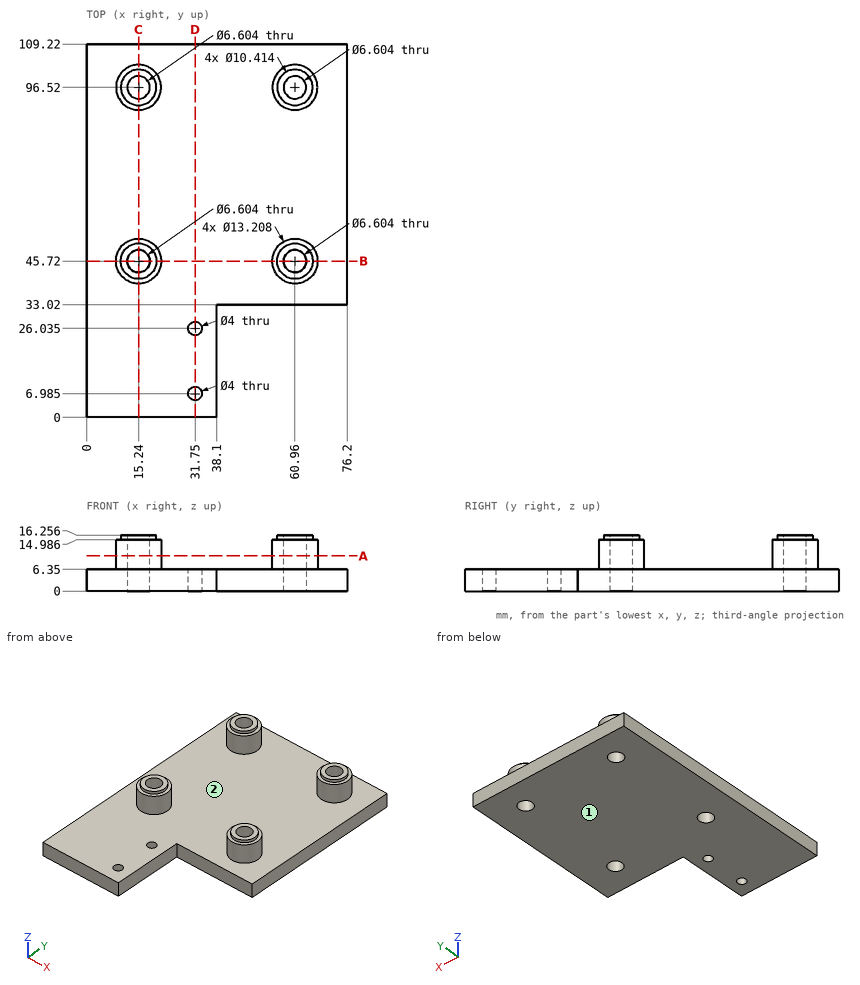
For this review, use the dimensioned drawing (mm, ordinates from the lowest corner) and the shaded views. Give positions to 0.01 mm unless a question says otherwise; leave off trailing zeros. Write each loop counter-clockwise with the first axis right and the second up, starting at its lowest first coordinate (ties: lowest second). Pieces come first, ordered by that corner, then holes. Notation, with made-up numbers: M 71,66 L 95,66 A27 ccw 95,88 Z; hole C -2.75,80 d11. An arc over 180 degrees is marked long. Answer as a JSON object with one key per item and string values. Group by question number.
1) For line 1 along Y through (x, z) = (60.96, 3.5); line 2 along Y through (x, z) = (60.96, 12.25); line 3 along X through (y, z) = (43.5, 4.25), list the stretches that pass through material, from the lowest coordinate up.
2) Mouldability with a two-part tool opening along Y and no side actions: class the marked faces 1 and 2 as released by +Y, released by -Y, zero draft, split by the parting line, or undercut.
3) Clearance check with flat-ended pins moving along their axes: pin 1 Ø6.5 at (x, y) = (31.75, 26.035) entering from +Z; pin 2 Ø8.5 at (x, y) = (60.96, 96.52) entering from -Z; pin 3 Ø8 at (x, z) = (60, 6.5) entering from -Y; pin 4 Ø7 at (y, z) = (17, 4) entering from +X. State where each tip first meets the part, or that it passes through.
4) We need section C-C (x = 15.24). Give the boundary of the cut face in (y, z).
5) We need section D-D (x = 31.75). Give the boundary of the cut face in (y, z) (3 decimals).
6) We need section B-B (y = 45.72). Give the boundary of the cut face in (x, z), and give its area (3 significant figures).
7) We need section A-A (z = 10.25). Give the boundary of the cut face in (x, y).
Answer key:
{
 "1": {"line 1": "y = 33.02 to 42.42, 49.02 to 93.22, 99.82 to 109.22", "line 2": "y = 39.12 to 42.42, 49.02 to 52.32, 89.92 to 93.22, 99.82 to 103.12", "line 3": "x = 0 to 12.8, 17.68 to 58.52, 63.4 to 76.2"},
 "2": {"face 1": "zero draft", "face 2": "undercut"},
 "3": {"pin 1": "stops at z = 6.35", "pin 2": "stops at z = 0", "pin 3": "stops at y = 33.02", "pin 4": "stops at x = 38.1"},
 "4": {"outline": "M 0,0 L 42.42,0 L 42.42,16.26 L 40.51,16.26 L 40.51,14.99 L 39.12,14.99 L 39.12,6.35 L 0,6.35 Z; M 49.02,0 L 93.22,0 L 93.22,16.26 L 91.31,16.26 L 91.31,14.99 L 89.92,14.99 L 89.92,6.35 L 52.32,6.35 L 52.32,14.99 L 50.93,14.99 L 50.93,16.26 L 49.02,16.26 Z; M 99.82,0 L 109.22,0 L 109.22,6.35 L 103.12,6.35 L 103.12,14.99 L 101.73,14.99 L 101.73,16.26 L 99.82,16.26 Z"},
 "5": {"outline": "M 0,0 L 4.985,0 L 4.985,6.35 L 0,6.35 Z; M 8.985,0 L 24.035,0 L 24.035,6.35 L 8.985,6.35 Z; M 28.035,0 L 109.22,0 L 109.22,6.35 L 28.035,6.35 Z"},
 "6": {"outline": "M 0,0 L 11.94,0 L 11.94,16.26 L 10.03,16.26 L 10.03,14.99 L 8.64,14.99 L 8.64,6.35 L 0,6.35 Z; M 18.54,0 L 57.66,0 L 57.66,16.26 L 55.75,16.26 L 55.75,14.99 L 54.36,14.99 L 54.36,6.35 L 21.84,6.35 L 21.84,14.99 L 20.45,14.99 L 20.45,16.26 L 18.54,16.26 Z; M 64.26,0 L 76.2,0 L 76.2,6.35 L 67.56,6.35 L 67.56,14.99 L 66.17,14.99 L 66.17,16.26 L 64.26,16.26 Z", "area": "524 mm²"},
 "7": {"outline": "C 15.24,45.72 d13.21; C 15.24,96.52 d13.21; C 60.96,45.72 d13.21; C 60.96,96.52 d13.21; hole C 15.24,45.72 d6.6; hole C 15.24,96.52 d6.6; hole C 60.96,45.72 d6.6; hole C 60.96,96.52 d6.6"}
}
